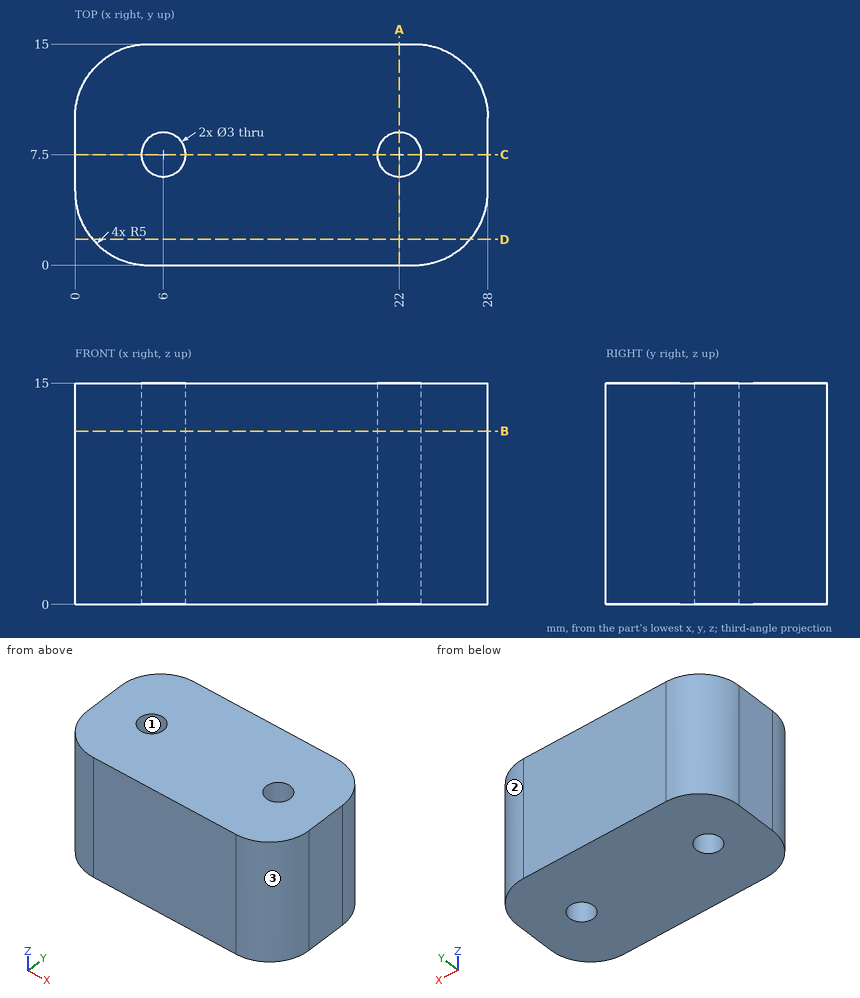
Source: three-view drawing plus pictorial views. Frame: mm from the lowest corner of the part. Give positions to 0.01 mm unless a question says otherwise; leave off trailing zeros. Order: outer loops, then holes, each group sorted by start corner. A loop starts at its lowest first (then second) coordinate and runs counter-clockwise, first axis right, second up. Notation, with made-up numbers: M 25,26.5 L 69,26.5 A16 cw 69,41.5 Z; hole C 76.25,59 d3. An arc over 180 degrees is marked long. Return JSON: item names as keys, results as strings.
1) Line query: L1, parallel to Y at x = 6, z = 10.5; L2, parallel to Y at x = 7, z = 6.5; L3, parallel to X at y = 12, z = 3. Output: solid intervals per line, ascending. Write a range as [from, to].
Taken from the geometry:
{"L1": "y = [0, 6], [9, 15]", "L2": "y = [0, 6.38], [8.62, 15]", "L3": "x = [0.42, 27.58]"}
2) Section query D-D on y = 1.75. Output: boundary loops of the cut face in (x, z).
Taken from the geometry:
{"outline": "M 1.2,0 L 26.8,0 L 26.8,15 L 1.2,15 Z"}
3) Section query B-B on z = 11.75. Output: boundary loops of the cut face in (x, y).
Taken from the geometry:
{"outline": "M 0,5 A5 ccw 5,0 L 23,0 A5 ccw 28,5 L 28,10 A5 ccw 23,15 L 5,15 A5 ccw 0,10 Z; hole C 6,7.5 d3; hole C 22,7.5 d3"}
4) Section query A-A on x = 22. Output: boundary loops of the cut face in (y, z).
Taken from the geometry:
{"outline": "M 0,0 L 6,0 L 6,15 L 0,15 Z; M 9,0 L 15,0 L 15,15 L 9,15 Z"}
5) Contact query for flat-ended pins moving along their axis: pin 1 (2.5 mm diameter, centred on x = 6, y = 7.5, fed in from -Z); pin 2 (1.5 mm diameter, centred on x = 24, z = 7.5, fed in from +Y). Output: stop coordinate, or through.
Taken from the geometry:
{"pin 1": "passes through", "pin 2": "stops at y = 14.99"}
6) Mould query, pull axis Y, two halves, no side actions, for the marked faces 1, 2 and 3. Classes: released by +Y, released by -Y, zero draft, split by the parting line, or undercut.
Taken from the geometry:
{"face 1": "undercut", "face 2": "released by +Y", "face 3": "released by -Y"}
7) Section query C-C on y = 7.5. Output: boundary loops of the cut face in (x, z), and give its area (3 significant figures).
Taken from the geometry:
{"outline": "M 0,0 L 4.5,0 L 4.5,15 L 0,15 Z; M 7.5,0 L 20.5,0 L 20.5,15 L 7.5,15 Z; M 23.5,0 L 28,0 L 28,15 L 23.5,15 Z", "area": "330 mm2"}
